from build123d import *

# Parameters (mm, degrees)
BOSS_EXTRUDE1_DEPTH = 16
SKETCH2_R           = 1.5
CUT_EXTRUDE1_DEPTH  = 84.837177911


with BuildPart() as part:
    # Sketch1 → Boss-Extrude1 (new body)
    with BuildSketch(Plane.XY):
        Polygon((0, 0), (0, 24), (8, 24), (8, 43), (16, 43), (16, 61.65), (25.77, 61.65), (25.77, 29.65), (55.27, 29.65), (55.27, 37.65), (67.12, 37.65), (67.12, 30.68), (75.82, 30.68), (75.82, 0), (57.7, 0), (57.7, 4), (20.5, 4), (20.5, 0), align=None)
    extrude(amount=BOSS_EXTRUDE1_DEPTH)

    # Sketch2 → Cut-Extrude1 (cut, through all)
    with BuildSketch(Plane(origin=(0, 29.65, 0), x_dir=(1, 0, 0), z_dir=(0, 1, 0))):
        with Locations(Location((47.57, -8, 0), (0, 0, 270))):
            Circle(SKETCH2_R)
    extrude(amount=-CUT_EXTRUDE1_DEPTH, mode=Mode.SUBTRACT)


solid = part.part
CAD build for the part. Positions are in the model's coordinates, mm. A direction names the side the tool comes from. Give positions to 0.01 mm unless a question says otherwise; leave off trailing zeros. Order: outer loops, then holes, each group sorted by start corner. A loop starts at its lowest first (then second) coordinate and runs counter-clockwise, first axis right, second up. Notation, with made-up numbers: (-24, 43.25) -> (7, 43.25) arc R26 cw to (7, 73.25) -> close; hole circle Ø3 at (-6.5, -8.5). An arc over 180 degrees is marked (long way). Return JSON: item names as keys, results as strings.
Q1. Which spindle directions (+Z, -Z, +X, -X, +Y, -Y) get a long thin tool onto all of the face, cutting with end or side? Do faces 4 (the face through (12, 43, 8)), 5 (the face through (61, 37.65, 8)), 6 (the face through (40, 29.65, 8)), 7 (the face through (57.7, 2, 8)). Say none if no direction does.
Working result:
{"face 4": "+Z, -Z, -X, +Y", "face 5": "+Z, -Z, +X, +Y", "face 6": "+Z, -Z, +Y", "face 7": "+Z, -Z, -Y"}
Q2. Mould opens along X. For faces 1 (the face through (8, 33, 8)), 2 (the face through (55.27, 34, 8)), 3 (the face through (38, 24, 0)) say: pulls with the +X half, pulls with the -X half, needs draft (parallel to the pull), parting line crosses it, or undercut.
Working result:
{"face 1": "pulls with the -X half", "face 2": "undercut", "face 3": "needs draft"}
Q3. Drill centre lines: line 1 (X direction, y = 16, z = 8); line 2 (X direction, y = 32, z = 7.5); line 3 (Y direction, x = 38, z = 13.75). Where is each one in solid material? Low to high.
Working result:
{"line 1": "0 to 46.07, 49.07 to 75.82", "line 2": "8 to 25.77, 55.27 to 67.12", "line 3": "4 to 29.65"}
Q4. Saw through at D-D (z = 3.5). Write the cut outline in (x, y).
Working result:
{"outline": "(0, 0) -> (20.5, 0) -> (20.5, 4) -> (57.7, 4) -> (57.7, 0) -> (75.82, 0) -> (75.82, 30.68) -> (67.12, 30.68) -> (67.12, 37.65) -> (55.27, 37.65) -> (55.27, 29.65) -> (25.77, 29.65) -> (25.77, 61.65) -> (16, 61.65) -> (16, 43) -> (8, 43) -> (8, 24) -> (0, 24) -> close"}
Q5. Saw through at B-B (y = 35.5). Write the cut outline in (x, z), then the cut area to 3 significant figures.
Working result:
{"outline": "(8, 0) -> (25.77, 0) -> (25.77, 16) -> (8, 16) -> close; (55.27, 0) -> (67.12, 0) -> (67.12, 16) -> (55.27, 16) -> close", "area": "474 mm²"}
Q6. Saw through at C-C (x = 47.57). Write the cut outline in (y, z), then the cut area to 3 significant figures.
Working result:
{"outline": "(4, 0) -> (29.65, 0) -> (29.65, 6.5) -> (4, 6.5) -> close; (4, 9.5) -> (29.65, 9.5) -> (29.65, 16) -> (4, 16) -> close", "area": "333 mm²"}
Q7. Flat gauge pins, fed straight in: pin 1 (1 mm diameter, centred on x = 60, y = 10.5, fed in from -Z); pin 2 (2.5 mm diameter, centred on y = 33, z = 10.5, fed in from -X); pin 3 (8 mm diameter, centred on x = 42.5, z = 4.5, fed in from +Y); pin 4 (7 mm diameter, centred on x = 71.5, z = 5, fed in from +Y). Where does each tip first touch, or does it go through?
Working result:
{"pin 1": "z = 0", "pin 2": "x = 8", "pin 3": "y = 29.65", "pin 4": "y = 30.68"}
Q8. Saw through at A-A (z = 8). Write the cut outline in (x, y).
Working result:
{"outline": "(0, 0) -> (20.5, 0) -> (20.5, 4) -> (46.07, 4) -> (46.07, 29.65) -> (25.77, 29.65) -> (25.77, 61.65) -> (16, 61.65) -> (16, 43) -> (8, 43) -> (8, 24) -> (0, 24) -> close; (49.07, 4) -> (57.7, 4) -> (57.7, 0) -> (75.82, 0) -> (75.82, 30.68) -> (67.12, 30.68) -> (67.12, 37.65) -> (55.27, 37.65) -> (55.27, 29.65) -> (49.07, 29.65) -> close"}
